```python
from build123d import *

# Parameters (mm, degrees)
F0_W = 76.2
F0_H = 12.7
F2_R = 19.05
F3_R = 12.7
F4_R = 12.69999
F5_R = 5.08
F6_R = 5.08


# Not quite as in the source:
# - a fillet or chamfer is up to 0.001 mm smaller than in the source, because OpenCascade refuses the exact size


with BuildPart() as f1:
    # F0 (on Front) → F1 (revolve)
    with BuildSketch(Plane.XZ):
        with Locations((-38.1, -180.2761299372)):
            Rectangle(F0_W, F0_H)
        Polygon((-76.2, -173.9261299372), (0, -173.9261299372), (0, 29.2738700628), (-12.7, 29.2738700628), (-76.2, 29.2738700628), align=None)
        Polygon((-12.7, 29.2738700628), (0, 29.2738700628), (0, 35.6238700628), (0, 41.9738700628), (-12.7, 41.9738700628), align=None)
        Polygon((-19.05, 41.9738700628), (-12.7, 41.9738700628), (0, 41.9738700628), (0, 61.0238700628), (0, 67.3738700628), (-19.05, 67.3738700628), align=None)
    revolve(axis=Axis((0, 0, -14.5017058273), (0, 0, -1)))

    # F2
    f2_edges = [f1.edges().sort_by_distance(p)[0] for p in [
        (76.2, 0, 29.27387),
    ]]
    fillet(f2_edges, radius=F2_R)

    # F3
    f3_edges = [f1.edges().sort_by_distance(p)[0] for p in [
        (76.2, 0, -186.62613),
    ]]
    fillet(f3_edges, radius=F3_R)

    # F4 (radius 12.7 in the source; OpenCascade refuses exactly that, so slightly less here)
    f4_edges = [f1.edges().sort_by_distance(p)[0] for p in [
        (12.7, 0, 29.27387),
    ]]
    fillet(f4_edges, radius=F4_R)

    # F5
    f5_edges = [f1.edges().sort_by_distance(p)[0] for p in [
        (19.05, 0, 41.97387),
    ]]
    fillet(f5_edges, radius=F5_R)

    # F6
    f6_edges = [f1.edges().sort_by_distance(p)[0] for p in [
        (19.05, 0, 67.37387),
    ]]
    fillet(f6_edges, radius=F6_R)


solid = f1.part
```
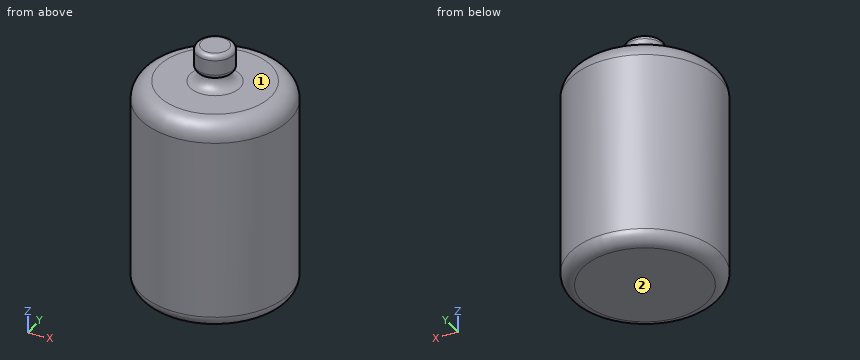
The listing builds one solid part. Answer for the finished solid, in the listing's coordinates (mm). Face numbers are marked on the shaded views. A direction names the side the tool comes from. Give positions to 0.01 mm unless a question says otherwise; leave off trailing zeros. Order: outer loops, then holes, each group sorted by start corner. A loop starts at its lowest first (then second) coordinate and runs counter-clockwise, first axis right, second up.
Item 1: Which of the six approach directions +Z, -Z, +X, -X, +Y, -Y give full straight-line access (tool end or side, diameter ignored) to the marked faces 1 and 2?
From the geometry:
face 1: +Z
face 2: -Z, +X, -X, +Y, -Y
Item 2: Given pin 1 Ø4 at (x, z) = (33.5, -112) entering from +Y; pin 2 Ø6 at (x, z) = (-23.5, -134) entering from +Y; pin 3 Ø1 at (x, y) = (36.5, 26) entering from +Z, each flat-ended and moving along its own axis, determine where each tip first touches the part or whether it passes through.
From the geometry:
pin 1: stops at y = 69.38
pin 2: stops at y = 73.39
pin 3: stops at z = 29.27
Item 3: The part is cut by section C-C, the plane z = -126.5. Give the vertices of the cut face in (x, y), and give its area (3 significant figures).
From the geometry:
outline: circle Ø152.4 at (0, 0)
area: 18,200 mm2
Item 4: Find the intervals of material crossed by probe 1 along Z at (x, y) = (43, 8); probe 2 along Y at (x, z) = (0.5, -125); probe 3 along X at (y, z) = (51, -35), in increasing order.
From the geometry:
probe 1: z = -186.63 to 29.27
probe 2: y = -76.2 to 76.2
probe 3: x = -56.62 to 56.62
